Check sheet for the modelled part. Datum: model origin and axes. Units: mm. A direction names the side the tool comes from. Coordinates: 2 decimals unless noted, no trailing zeros. Order: outer loops, then holes, each group sorted by start corner. A loop starts at its lowest first (then second) coordinate and runs counter-clockwise, first axis right, second up. Notation, with made-up numbers: (-23, 26.25) -> (32, 26.25) arc R8 cw to (32, 39.25) -> close; hole circle Ø6 at (22, 20.5). An arc over 180 degrees is marked (long way). Put each result on its own line as item: value. Start each with the question number.
```python
from build123d import *

# Parameters (mm, degrees)
F0_R           = 13.5
F1_DEPTH       = 64
F2_W           = 102
F2_H           = 13
F3_DEPTH       = 400
F5_DEPTH       = 13
F7_DEPTH       = 13
F8_R           = 15
F9_DEPTH       = 43
F14_DEPTH      = 3.5
F14_DEPTH_BACK = 3.5
F15_R          = 8
F16_DEPTH      = 25
F17_T4_DEPTH   = 101.551131953
F17_S5_R       = 20
F17_T6_DEPTH   = 53
F17_T10_DEPTH  = 101.551131953
F17_S11_R      = 20
F17_T12_DEPTH  = 53
F17_T16_DEPTH  = 50.1219672703
F17_S17_R      = 15
F17_T18_DEPTH  = 28
F17_T22_DEPTH  = 50.1219672703
F17_S23_R      = 15
F17_T24_DEPTH  = 28


# Not quite as in the source:
# - a fillet or chamfer that OpenCascade refuses, or shapes differently, is made with other operations: its cross-section is extruded or revolved along the edge and cut away or added


with BuildPart() as f1:
    # F0 (on Front) → F1 (new body)
    with BuildSketch(Plane.XZ):
        with BuildLine():
            Line((-7, -214.9833835959), (0, -214.9833835959))
            Line((0, -214.9833835959), (0, -101.8451102358))
            ThreePointArc((0, -101.8451102358), (-0.1689225963, -100.0148323657), (-0.6699834164, -98.2463895535))
            Line((-0.6699834164, -98.2463895535), (-26.3300165836, -31.7203776383))
            ThreePointArc((-26.3300165836, -31.7203776383), (-26.8310774037, -29.9519348262), (-27, -28.1216569561))
            Line((-27, -28.1216569561), (-27, 80.0166164041))
            ThreePointArc((-27, 80.0166164041), (-28.4644660941, 83.55215031), (-32, 85.0166164041))
            Line((-32, 85.0166164041), (-102, 85.0166164041))
            ThreePointArc((-102, 85.0166164041), (-141.2677104995, 91.7114873793), (-103.8614958525, 78.0166164041))
            Line((-103.8614958525, 78.0166164041), (-39, 78.0166164041))
            ThreePointArc((-39, 78.0166164041), (-35.4644660941, 76.55215031), (-34, 73.0166164041))
            Line((-34, 73.0166164041), (-34, -28.1216569561))
            ThreePointArc((-34, -28.1216569561), (-33.8310774037, -29.9519348262), (-33.3300165836, -31.7203776383))
            Line((-33.3300165836, -31.7203776383), (-7.6699834164, -98.2463895535))
            ThreePointArc((-7.6699834164, -98.2463895535), (-7.1689225963, -100.0148323657), (-7, -101.8451102358))
            Line((-7, -101.8451102358), (-7, -214.9833835959))
        make_face()
        with Locations((-121.9394617303, 86.5715652479)):
            Circle(F0_R, mode=Mode.SUBTRACT)
    extrude(amount=F1_DEPTH)

    # F2 (on face) → F3 (cut)
    with BuildSketch(Plane.XY.offset(85.0166164041)):
        with Locations((-51, -6.5)):
            Rectangle(F2_W, F2_H)
        with Locations((-51, -57.5)):
            Rectangle(F2_W, F2_H)
    extrude(amount=-F3_DEPTH, mode=Mode.SUBTRACT)

    # F4 (on face) → F5 (cut)
    with BuildSketch(Plane(origin=(0, 0, 0), x_dir=(-1, 0, 0), z_dir=(0, 1, 0))):
        with BuildLine():
            ThreePointArc((103.8614958525, 78.0166164041), (102.6112129611, 81.4316431166), (102, 85.0166164041))
            Line((102, 85.0166164041), (102, 78.0166164041))
            Line((102, 78.0166164041), (103.8614958525, 78.0166164041))
        make_face()
    extrude(amount=-F5_DEPTH, mode=Mode.SUBTRACT)

    # F6 (on face) → F7 (cut)
    with BuildSketch(Plane.XZ.offset(64)):
        with BuildLine():
            Line((-102, 78.0166164041), (-102, 85.0166164041))
            ThreePointArc((-102, 85.0166164041), (-102.6112129611, 81.4316431166), (-103.8614958525, 78.0166164041))
            Line((-103.8614958525, 78.0166164041), (-102, 78.0166164041))
        make_face()
    extrude(amount=-F7_DEPTH, mode=Mode.SUBTRACT)

    # F8 (on face) → F9 (join)
    with BuildSketch(Plane.YZ.offset(-27)):
        with Locations((-32, 55.0166164041)):
            Circle(F8_R)
    extrude(amount=F9_DEPTH)

    # F11 (on face) → F12 (revolve)
    with BuildSketch(Plane(origin=(0, -32, 0), x_dir=(-1, 0, 0), z_dir=(0, 1, 0))):
        Polygon((-16, 55.0166164041), (-16, 70.0166164041), (-19, 68.0166164041), (-19, 65.0166164041), (-42, 65.0166164041), (-43, 63.5166164041), (-43, 55.0166164041), align=None)
    revolve(axis=Axis((29.5, -32, 55.0166164041), (1, 0, 0)))

    # F13 (on face) → F14 (join, two sides)
    with BuildSketch(Plane(origin=(0, -32, 0), x_dir=(-1, 0, 0), z_dir=(0, 1, 0))) as f14_sk:
        with BuildLine():
            ThreePointArc((102.0563293248, 85.0166164041), (104.6045567862, 96.385687049), (113.0563293248, 104.4054608288))
            Line((113.0563293248, 104.4054608288), (29.0563293248, 97.8962504797))
            Line((29.0563293248, 97.8962504797), (13.0563293248, 70.0166164041))
            Line((13.0563293248, 70.0166164041), (10.7852649025, 66.0593385881))
            Line((10.7852649025, 66.0593385881), (27, 66.0593385881))
            Line((27, 66.0593385881), (27, 70.0166164041))
            Line((27, 70.0166164041), (27, 80.0166164041))
            ThreePointArc((27, 80.0166164041), (28.4644660941, 83.55215031), (32, 85.0166164041))
            Line((32, 85.0166164041), (102.0563293248, 85.0166164041))
        make_face()
    extrude(amount=F14_DEPTH)
    extrude(f14_sk.sketch, amount=-F14_DEPTH_BACK)

    # F15 (on face) → F16 (cut)
    with BuildSketch(Plane.YZ):
        with Locations((-32, -196.9833835959)):
            Circle(F15_R)
    extrude(amount=-F16_DEPTH, mode=Mode.SUBTRACT)

    # F17: fillet of radius 3.5 on 4 edges, made by hand


with BuildPart() as f17_tool2:
    # F17_s3 → F17_t4 (new body)
    with BuildSketch(Plane(origin=(-128.9474066936, 0, 9.992211835), x_dir=(0, 1, 0), z_dir=(0.9970110578, 0, -0.0772589845))):
        with BuildLine():
            ThreePointArc((-35.5, 91.8587817466), (-34.4748737342, 94.3336554808), (-32, 95.3587817466))
            Line((-32, 95.3587817466), (-35.5, 95.3587817466))
            Line((-35.5, 95.3587817466), (-35.5, 91.8587817466))
        make_face()
    extrude(amount=F17_T4_DEPTH)

    # F17_s5 → F17_t6 (cut, symmetric)
    with BuildSketch(Plane.XZ.offset(33.8)):
        with Locations((-121.9394617303, 86.5715652479)):
            Circle(F17_S5_R)
    extrude(amount=F17_T6_DEPTH, both=True, mode=Mode.SUBTRACT)


with BuildPart() as f1_1:
    add(f1.part)

    # F17_t1: cut F17_tool2
    add(f17_tool2.part, mode=Mode.SUBTRACT)


with BuildPart() as f17_tool8:
    # F17_s9 → F17_t10 (new body)
    with BuildSketch(Plane(origin=(-128.9474066936, 0, 9.992211835), x_dir=(0, 1, 0), z_dir=(0.9970110578, 0, -0.0772589845))):
        with BuildLine():
            ThreePointArc((-28.5, 91.8587817466), (-29.5251262658, 94.3336554808), (-32, 95.3587817466))
            Line((-32, 95.3587817466), (-28.5, 95.3587817466))
            Line((-28.5, 95.3587817466), (-28.5, 91.8587817466))
        make_face()
    extrude(amount=F17_T10_DEPTH)

    # F17_s11 → F17_t12 (cut, symmetric)
    with BuildSketch(Plane.XZ.offset(30.2)):
        with Locations((-121.9394617303, 86.5715652479)):
            Circle(F17_S11_R)
    extrude(amount=F17_T12_DEPTH, both=True, mode=Mode.SUBTRACT)


with BuildPart() as f1_2:
    add(f1_1.part)

    # F17_t7: cut F17_tool8
    add(f17_tool8.part, mode=Mode.SUBTRACT)


with BuildPart() as f17_tool14:
    # F17_s15 → F17_t16 (new body)
    with BuildSketch(Plane(origin=(-53.8169429454, 0, 93.7747922742), x_dir=(0, 1, 0), z_dir=(0.4977511049, 0, -0.8673199165))):
        with BuildLine():
            ThreePointArc((-35.5, 20.026833714), (-34.4748737342, 22.5017074481), (-32, 23.526833714))
            Line((-32, 23.526833714), (-35.5, 23.526833714))
            Line((-35.5, 23.526833714), (-35.5, 20.026833714))
        make_face()
    extrude(amount=F17_T16_DEPTH)

    # F17_s17 → F17_t18 (cut, symmetric)
    with BuildSketch(Plane.YZ.offset(-22.5)):
        with Locations((-32, 55.0166164041)):
            Circle(F17_S17_R)
    extrude(amount=F17_T18_DEPTH, both=True, mode=Mode.SUBTRACT)


with BuildPart() as f1_3:
    add(f1_2.part)

    # F17_t13: cut F17_tool14
    add(f17_tool14.part, mode=Mode.SUBTRACT)


with BuildPart() as f17_tool20:
    # F17_s21 → F17_t22 (new body)
    with BuildSketch(Plane(origin=(-28.8686783585, 0, 50.3030118051), x_dir=(0, 1, 0), z_dir=(-0.4977511049, 0, 0.8673199165))):
        with BuildLine():
            ThreePointArc((-28.5, -20.026833714), (-29.5251262658, -22.5017074481), (-32, -23.526833714))
            Line((-32, -23.526833714), (-28.5, -23.526833714))
            Line((-28.5, -23.526833714), (-28.5, -20.026833714))
        make_face()
    extrude(amount=F17_T22_DEPTH)

    # F17_s23 → F17_t24 (cut, symmetric)
    with BuildSketch(Plane.YZ.offset(-22.5)):
        with Locations((-32, 55.0166164041)):
            Circle(F17_S23_R)
    extrude(amount=F17_T24_DEPTH, both=True, mode=Mode.SUBTRACT)


with BuildPart() as f1_4:
    add(f1_3.part)

    # F17_t19: cut F17_tool20
    add(f17_tool20.part, mode=Mode.SUBTRACT)


solid = f1_4.part
```
1) Scan lines: line 1 along X through (y, z) = (-45, -129); line 2 along X through (y, z) = (-31, -19); line 3 along Y through (x, z) = (-40.5, 91). Record each from-to range of solid material in increasing order. Write a range as [from, to].
2) Mould release check, pull along Y, two halves, no side actions. Record for faces 5 (the cylindrical face through (30.66, -23.13, 59.63)), 6 (the cylindrical face through (-3.5, -33.7, -204.8)), 7 (the flat face through (-109, -64, 82)): +Y half, -Y half, draft (parallel to the pull), parting line (faces both ways), or undercut.
3) Sectioned sample at B-B (x = 9). Record the boundary of the cut face in (y, z).
4) Access from +Z, -Z, +X, -X, +Y, -Y to the whole of each face (thin tool, end or side, straight path). Record for faces 1 (the flat face through (-67, -21, 85.017)), 2 (the flat face through (-67, -43, 85.017)), 3 (the flat face through (-13.32, -31.73, -65.45)), 4 (the flat face through (-72, -32, 78.017)).
5) Sectioned sample at A-A (y = -6). Record the boundary of the cut face in (x, z), plus the area to 3 significant figures.
6) Gauge pin test, flat ends, axial feed: pin 1 (9.5 mm diameter, centred on x = -76, z = 91, fed in from -Y); pin 2 (1 mm diameter, centred on y = -52.5, z = -36.5, fed in from +X); pin 3 (24.5 mm diameter, centred on x = -40.5, z = 91.5, fed in from +Y); pin 4 (17 mm diameter, centred on x = -76, y = -40.5, fed in from +Z). Record the tip position at first contact, or that the pin passes through.
Entries:
1. line 1: x = [-7, 0]
1. line 2: x = [-34, -27]
1. line 3: y = [-35.5, -28.5]
2. face 5: parting line
2. face 6: undercut
2. face 7: -Y half
3. outline: circle Ø30 at (-32, 55.02)
4. face 1: +Z, +X, +Y
4. face 2: +Z, +X, -Y
4. face 3: +X, +Y, -Y
4. face 4: -Z, +Y, -Y
5. outline: circle Ø40 at (-121.94, 86.57); hole circle Ø27 at (-121.94, 86.57)
5. area: 684 mm2
6. pin 1: stops at y = -35.5
6. pin 2: passes through
6. pin 3: stops at y = -13
6. pin 4: stops at z = 101.73
